Can you work these out from the drawing? Everything is in mm from the part's minimum corner. A direction names the side the tool comes from. Coordinates: 2 decimals unless noted, no trailing zeros. Order: outer loops, then holes, each group sorted by start corner. A loop starts at its lowest first (then second) coordinate and runs counter-clockwise, first axis right, second up. Notation, with made-up numbers: (59, 41) -> (96, 41) arc R18 ccw to (96, 58) -> close; hole circle Ø3 at (43.5, 87.5). An arc over 180 degrees is marked (long way). Return JSON: item names as keys, results as strings. Group by question number.
1) If we section it at C-C, the plane x = 317.5: Please give me the cut outline in (y, z) (1 decimal), then the cut area to 3 significant figures.
2) Thinking about a two-plate mould opening in Y: for the marked faces 4, 5 and 6, which applies, +Y half, -Y half, draft (parallel to the pull), parting line (faces both ways), or undercut?
3) For the marked faces 1, 2 and 3, which set-ups out of +Z, -Z, +X, -X, +Y, -Y let a thin tool reach every point of the face, with its end or its side?
4) If we section it at D-D, the plane y = 69.5: Please give me the cut outline in (x, z).
5) For pin 1 (10 mm diameter, centred on x = 409.5, z = 72, fed in from -Y); pin 2 (1.5 mm diameter, centred on x = 270, z = 157.5, fed in from +Y); pin 3 (2 mm diameter, centred on x = 314, y = 130.5, fed in from +Z); pin 4 (1.5 mm diameter, centred on y = 102.5, z = 228.5, fed in from -X), each with a flat end and sliding along its axis, tell me the tip position at first contact or that it passes through.
6) If I drill on probe 1 along Y at (x, z) = (593, 45.5); probe 2 along X at (y, z) = (103.5, 63) (1 decimal); probe 3 along Y at (x, z) = (312.5, 210), over which ranges is the centre line in solid material (lowest first)? Write a range as from..to.
7) If we section it at B-B, the plane z = 106: Please give me the cut outline in (x, y) (1 decimal).
8) If we section it at A-A, the plane y = 36: Please give me the cut outline in (x, z).
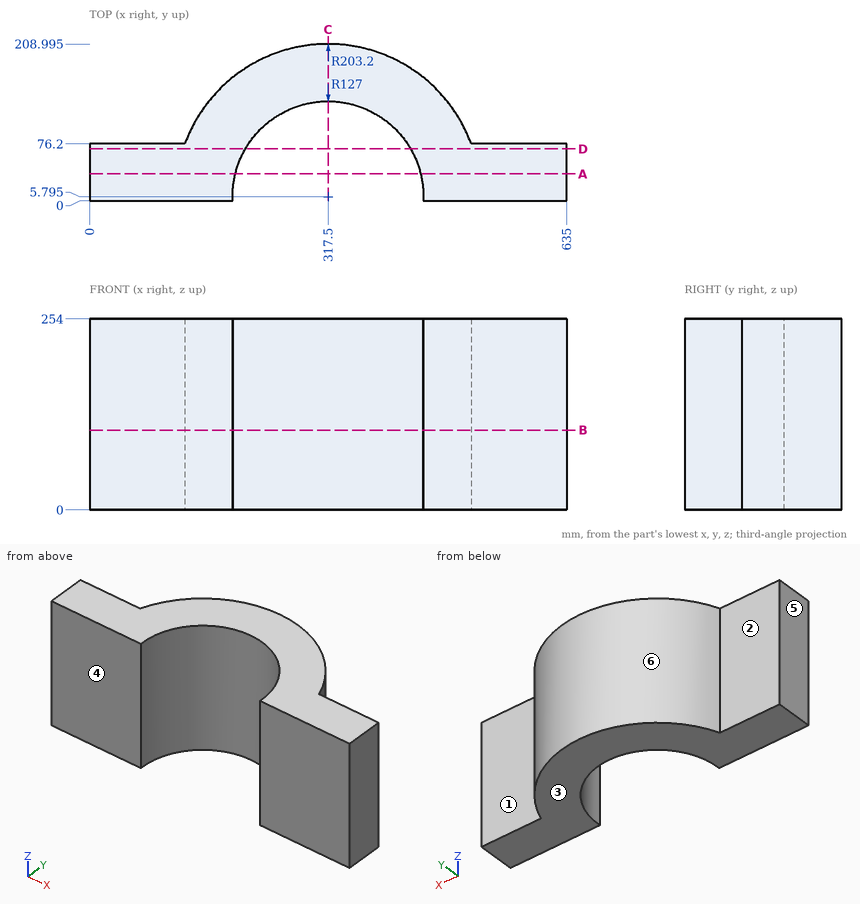
Result sheet:
{
 "1": {"outline": "(132.8, 0) -> (209, 0) -> (209, 254) -> (132.8, 254) -> close", "area": "19,400 mm2"},
 "2": {"face 4": "-Y half", "face 5": "draft", "face 6": "+Y half"},
 "3": {"face 1": "+Z, -Z, +X, +Y", "face 2": "+Z, -Z, -X, +Y", "face 3": "-Z, +X, -X, +Y, -Y"},
 "4": {"outline": "(0, 0) -> (207.63, 0) -> (207.63, 254) -> (0, 254) -> close; (427.37, 0) -> (635, 0) -> (635, 254) -> (427.37, 254) -> close"},
 "5": {"pin 1": "stops at y = 87.77", "pin 2": "stops at y = 203.54", "pin 3": "passes through", "pin 4": "stops at x = 138.38"},
 "6": {"probe 1": "y = 0..76.2", "probe 2": "x = 139.3..236.4, 398.6..495.7", "probe 3": "y = 132.7..208.93"},
 "7": {"outline": "(0, 0) -> (190.6, 0) arc R127 cw (long way) to (444.4, 0) -> (635, 0) -> (635, 76.2) -> (508.1, 76.2) arc R203.2 ccw to (126.9, 76.2) -> (0, 76.2) -> close"},
 "8": {"outline": "(0, 0) -> (194.14, 0) -> (194.14, 254) -> (0, 254) -> close; (440.86, 0) -> (635, 0) -> (635, 254) -> (440.86, 254) -> close"}
}
